from build123d import *

# Parameters (mm, degrees)
SKETCH_1_W                       = 540
SKETCH_1_H                       = 4
SM_BASE_FLANGE_1_DEPTH           = 100
SM_EDGE_FLANGE_1_STRIP_W         = 17.5
SM_EDGE_FLANGE_1_STRIP_H         = 4
SM_EDGE_FLANGE_1_STRIP_CUT_DEPTH = 100
SM_EDGE_FLANGE_1_DEPTH           = 100


# Sheet-metal steps are written as plain solids
with BuildPart() as part:
    # Sketch 1 → Базовая кромка1 (new body)
    with BuildSketch(Plane(origin=(0, 0, 0), x_dir=(1, 0, 0), z_dir=(0, 1, 0))):
        with Locations((270, -4)):
            Rectangle(SKETCH_1_W, SKETCH_1_H)
    extrude(amount=-SM_BASE_FLANGE_1_DEPTH)

    # Ребро-кромка1 strip (across the edge) → Ребро-кромка1 strip cut (cut)
    with BuildSketch(Plane(origin=(540, 0, 2), x_dir=(-1, 0, 0), z_dir=(0, -1, 0))):
        with Locations((-4, -2)):
            Rectangle(SM_EDGE_FLANGE_1_STRIP_W, SM_EDGE_FLANGE_1_STRIP_H)
    extrude(amount=SM_EDGE_FLANGE_1_STRIP_CUT_DEPTH, mode=Mode.SUBTRACT)

    # Ребро-кромка1 section (across the edge) → Ребро-кромка1 (add)
    with BuildSketch(Plane(origin=(540, 0, 2), x_dir=(-1, 0, 0), z_dir=(0, -1, 0))):
        with BuildLine():
            Line((0, 0.75), (0, 21))
            Line((0, 21), (4, 21))
            Line((4, 21), (4, 0.75))
            ThreePointArc((4, 0.75), (4.219669914, 0.219669914), (4.75, 0))
            Line((4.75, 0), (4.75, -4))
            ThreePointArc((4.75, -4), (1.391242789, -2.608757211), (0, 0.75))
        make_face()
    extrude(amount=SM_EDGE_FLANGE_1_DEPTH)

    # Зеркальное отражение1: part across plane


with BuildPart() as part_1:
    add(part.part)
    add(part.part.mirror(Plane(origin=(0, 0, 0), x_dir=(0, 0, 1), z_dir=(0, -1, 0))))

    # Зеркальное отражение2: part across face


with BuildPart() as part_2:
    add(part_1.part)
    add(part_1.part.mirror(Plane(origin=(0, 0, 4), x_dir=(0, 0, 1), z_dir=(-1, 0, 0))))


solid = part_2.part
Verification items for the finished model (mm, model axes). A direction names the side the tool comes from. Coordinates: 2 decimals unless noted, no trailing zeros. Order: outer loops, then holes, each group sorted by start corner. A loop starts at its lowest first (then second) coordinate and runs counter-clockwise, first axis right, second up.
1. Sectioned sample at C-C, the plane x = -113. Record the cut outline in (y, z), and give its area (3 significant figures).
Results found:
outline: (-100, 2) - (100, 2) - (100, 6) - (-100, 6) - close
area: 800 mm2
2. Release check for a two-part mould opening along X. For faces 1 (the face through (-540, -1, -9)), 2 (the face through (536, -1, -9)), 3 (the face through (7, -1, 6)) record: +X half, -X half, draft (parallel to the pull), parting line (faces both ways), or undercut.
Results found:
face 1: -X half
face 2: undercut
face 3: draft
3. Set-up check for faces 4 (the face through (3, 100, 4)), 5 (the face through (-536, -1, -9)): record each of +Z, -Z, +X, -X, +Y, -Y from which the full face is reachable in a straight line by a thin tool's end or side.
Results found:
face 4: +Z, -Z, +X, -X, +Y
face 5: -Z, +Y, -Y
4. Sectioned sample at B-B, the plane y = -1.5. Record the cut outline in (x, z), and give its area (3 significant figures).
Results found:
outline: (-540, -19) - (-536, -19) - (-536, 1.25) arc R0.75 cw to (-535.25, 2) - (535.25, 2) arc R0.75 cw to (536, 1.25) - (536, -19) - (540, -19) - (540, 1.25) arc R4.75 ccw to (535.25, 6) - (-535.25, 6) arc R4.75 ccw to (-540, 1.25) - close
area: 4,480 mm2
5. Scan lines: line 1 (X direction, y = 92.5, z = -5); line 2 (Z direction, x = 375, y = 28.5); line 3 (X direction, y = -25, z = 3.25). Record each from-to range of solid material in increasing order.
Results found:
line 1: x = -540 to -536, 536 to 540
line 2: z = 2 to 6
line 3: x = -539.56 to 539.56
6. Sectioned sample at A-A, the plane z = -9.5. Record the cut outline in (x, y), and give its area (3 significant figures).
Results found:
outline: (-540, -100) - (-536, -100) - (-536, 100) - (-540, 100) - close; (536, -100) - (540, -100) - (540, 100) - (536, 100) - close
area: 1,600 mm2
